Source: CAD feature listing. Evaluate the final solid. Frame: model axes, mm. A direction names the side the tool comes from. Round coordinates to 2 decimals unless told otherwise and drop trailing zeros. Order: outer loops, then holes, each group sorted by start corner. A loop starts at its lowest first (then second) coordinate and runs counter-clockwise, first axis right, second up. Notation, with made-up numbers: M 66,64 L 106,64 A32 cw 106,101 Z; hole C 89.25,13.5 d4. An arc over 180 degrees is marked long. Answer in a Markdown table with one row per item. Add a question column.
```python
from build123d import *

# Parameters (mm, degrees)
SKETCH1_R           = 1.65
BOSS_EXTRUDE1_DEPTH = 3
SKETCH3_W           = 11
SKETCH3_H           = 6
CUT_EXTRUDE2_DEPTH  = 1.2
SKETCH4_R           = 1.65
BOSS_EXTRUDE2_DEPTH = 2.8


with BuildPart() as part:
    # Sketch1 → Boss-Extrude1 (new body)
    with BuildSketch(Plane(origin=(0, 0, 0), x_dir=(0, 0, -1), z_dir=(1, 0, 0))):
        with BuildLine():
            Line((0, 3), (40.5, 3))
            ThreePointArc((40.5, 3), (43.5, 0), (40.5, -3))
            Line((40.5, -3), (0, -3))
            ThreePointArc((0, -3), (-3, 0), (0, 3))
        make_face()
        Circle(SKETCH1_R, mode=Mode.SUBTRACT)
        with Locations((40.5, 0)):
            Circle(SKETCH1_R, mode=Mode.SUBTRACT)
    extrude(amount=BOSS_EXTRUDE1_DEPTH)

    # Sketch3 → Cut-Extrude2 (cut)
    with BuildSketch(Plane.ZY):
        with Locations((-38, 0)):
            Rectangle(SKETCH3_W, SKETCH3_H)
    extrude(amount=-CUT_EXTRUDE2_DEPTH, mode=Mode.SUBTRACT)

    # Sketch4 → Boss-Extrude2 (add)
    with BuildSketch(Plane(origin=(3, 0, 0), x_dir=(0, 0, -1), z_dir=(1, 0, 0))):
        with BuildLine():
            Line((40.5, 3), (23.5, 3))
            Line((23.5, 3), (23.5, -3))
            Line((23.5, -3), (40.5, -3))
            ThreePointArc((40.5, -3), (43.5, 0), (40.5, 3))
        make_face()
        with Locations((40.5, 0)):
            Circle(SKETCH4_R, mode=Mode.SUBTRACT)
    extrude(amount=BOSS_EXTRUDE2_DEPTH)


solid = part.part
```
(1) Cut plane B-B (y = 0). Return loops of the section in (x, z), and give its area (3 significant figures).
(2) Cut plane C-C (z = -40). Return loops of the section in (x, y).
(3) Cut plane D-D (z = -13.5). Return loops of the section in (x, y), and give its area (3 significant figures).
(4) Access query for faces 1 (the face through (1, 0, -32.5)), 2 (the face through (4, 0, -23.5)), 3 (the face through (2, 3, -21)). Directions: +Z, -Z, +X, -X, +Y, -Y. A direction counts if a zero-diameter tool reaches every point of the face in a straight line with its end or side. Return the directions, or none.
(5) Cut plane A-A (x = 0.6). Return loops of the section in (y, z), and give its area (3 significant figures).
(6) Draft query along Z for faces 4 (the face through (1.479, 1.115, 1.216)), 5 (the face through (3.5, -0.1, -43.5)), 6 (the face through (2, -3, -20)). Return one class per face: +Z half, -Z half, draft (parallel to the pull), parting line (faces both ways), or undercut.
(7) Line query: line 1 (Y direction, x = 1.85, z = 0); line 2 (Z direction, x = 3.05, y = 0); line 3 (X direction, y = -1.25, z = -16). Output: solid intervals per line, ascending. Write a range as from..to.
(8) Pin query (flat end, axial travel): pin 1 (1 mm diameter, centred on y = 1.5, z = -10, fed in from +X); pin 2 (2 mm diameter, centred on y = 0, z = -40.5, fed in from +X); pin 3 (1.8 mm diameter, centred on y = 0.5, z = -36.5, fed in from -X). Return the tip coordinate at first contact, or that it passes through.
Answer list:
| question | item | result |
|---|---|---|
| 1 | outline | M 0,-32.5 L 1.2,-32.5 L 1.2,-38.85 L 5.8,-38.85 L 5.8,-23.5 L 3,-23.5 L 3,-1.65 L 0,-1.65 Z; M 0,1.65 L 3,1.65 L 3,3 L 0,3 Z; M 1.2,-43.5 L 5.8,-43.5 L 5.8,-42.15 L 1.2,-42.15 Z |
| 1 | area | 157 mm² |
| 2 | outline | M 1.2,-3 L 5.8,-3 L 5.8,-1.57 L 1.2,-1.57 Z; M 1.2,1.57 L 5.8,1.57 L 5.8,3 L 1.2,3 Z |
| 3 | outline | M 0,-3 L 3,-3 L 3,3 L 0,3 Z |
| 3 | area | 18.0 mm² |
| 4 | face 1 | -Z, -X, +Y, -Y |
| 4 | face 2 | +Z, +X, +Y, -Y |
| 4 | face 3 | +Z, -Z, +X, -X, +Y |
| 5 | outline | M -3,-32.5 L 3,-32.5 L 3,0 A3 ccw -3,0 Z; hole C 0,0 d3.3 |
| 5 | area | 201 mm² |
| 6 | face 4 | undercut |
| 6 | face 5 | -Z half |
| 6 | face 6 | draft |
| 7 | line 1 | -3..-1.65, 1.65..3 |
| 7 | line 2 | -43.5..-42.15, -38.85..-23.5 |
| 7 | line 3 | 0..3 |
| 8 | pin 1 | x = 3 |
| 8 | pin 2 | through |
| 8 | pin 3 | x = 1.2 |
